Input: part model. Units: mm. Frame: model coordinates. Face numbers are marked on the shaded views. A direction names the side the tool comes from. Round coordinates to 2 decimals unless told otherwise and drop trailing zeros. Loops run counter-clockwise (first coordinate to the right, second up) from the corner with the lowest first, then second, coordinate; pieces in that order, holes last. Notation, with made-up numbers: (10.5, 80.25) -> (42.5, 80.25) arc R16 ccw to (42.5, 110.25) -> close; hole circle Ø1 at (16, 30.5). An arc over 180 degrees is marked (long way). Answer in a Markdown table with one row per item. Add a question column.
Q1. Ray query, L1, parallel to X at y = -20.25, z = 0.25; L2, parallel to X at y = -4, z = -2.25; L3, parallel to Z at x = 2.25, y = -18.5. Return the intervals inside material, ascending. Write a range as from..to.
Q2. Section B-B, the plane x = 4. Output: boundary loops of the cut face in (y, z), and give its area (3 significant figures).
Q3. Mould query, pull axis Z, two halves, no side actions, for the marked faces 3, 4 and 5. Classes: pulls with the +Z half, pulls with the -Z half, needs draft (parallel to the pull), parting line crosses it, or undercut.
Q4. Section A-A, the plane z = 2.75. Output: boundary loops of the cut face in (x, y).
Q5. Section D-D, the plane z = -8. Output: boundary loops of the cut face in (x, y).
Q6. Reachability of the marked faces 1 and 2 from +Z, -Z, +X, -X, +Y, -Y: full face, straight path, thin tool, end or side. Return the list, or none.
Q7. Pin query (flat end, axial travel): pin 1 (2 mm diameter, centred on y = -16.5, z = -3, fed in from +X); pin 2 (5 mm diameter, centred on x = -3, y = -12.5, fed in from -Z); pin 3 (1.7 mm diameter, centred on y = -2, z = 1, fed in from -X); pin 4 (4 mm diameter, centred on x = -1, z = -2.5, fed in from +Y). Return the tip coordinate at first contact, or that it passes through.
```python
from build123d import *

# Parameters (mm, degrees)
F0_R     = 9.525
F1_DEPTH = 25.4
F3_DEPTH = 25.401
F4_DEPTH = 5.5499


with BuildPart() as f1:
    # F0 (on Front) → F1 (new body)
    with BuildSketch(Plane.XZ):
        Circle(F0_R)
    extrude(amount=F1_DEPTH)

    # F2 (on Front) → F3 (cut, through all)
    with BuildSketch(Plane.XZ):
        with BuildLine():
            ThreePointArc((4.7625, 0), (3.367596, 3.367596), (0, 4.7625))
            ThreePointArc((0, 4.7625), (-3.367596, 3.367596), (-4.7625, 0))
            ThreePointArc((-4.7625, 0), (-3.367596, -3.367596), (0, -4.7625))
            ThreePointArc((0, -4.7625), (3.367596, -3.367596), (4.7625, 0))
        make_face()
    extrude(amount=F3_DEPTH, mode=Mode.SUBTRACT)

    # F2 (on Front) → F4 (cut, symmetric)
    with BuildSketch(Plane.XZ):
        with BuildLine():
            Line((0, 4.7625), (-4.7625, 4.7625))
            Line((-4.7625, 4.7625), (-4.7625, 0))
            ThreePointArc((-4.7625, 0), (-3.367596, 3.367596), (0, 4.7625))
        make_face()
        with BuildLine():
            Line((4.7625, 4.7625), (0, 4.7625))
            ThreePointArc((0, 4.7625), (3.367596, 3.367596), (4.7625, 0))
            Line((4.7625, 0), (4.7625, 4.7625))
        make_face()
        with BuildLine():
            ThreePointArc((0, -4.7625), (-3.367596, -3.367596), (-4.7625, 0))
            Line((-4.7625, 0), (-4.7625, -4.7625))
            Line((-4.7625, -4.7625), (0, -4.7625))
        make_face()
        with BuildLine():
            Line((4.7625, -4.7625), (4.7625, 0))
            ThreePointArc((4.7625, 0), (3.367596, -3.367596), (0, -4.7625))
            Line((0, -4.7625), (4.7625, -4.7625))
        make_face()
    extrude(amount=F4_DEPTH, both=True, mode=Mode.SUBTRACT)


solid = f1.part
```
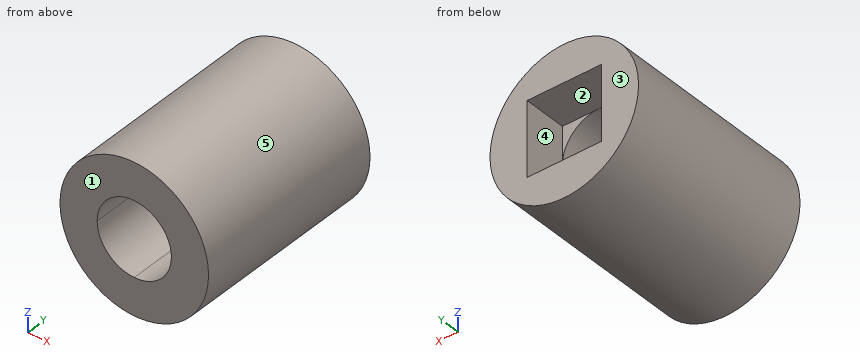
Answer block:
| question | item | result |
|---|---|---|
| 1 | L1 | -9.52..-4.76, 4.76..9.52 |
| 1 | L2 | -9.26..-4.76, 4.76..9.26 |
| 1 | L3 | -9.26..-4.2, 4.2..9.26 |
| 2 | outline | (-25.4, -8.64) -> (0, -8.64) -> (0, -4.76) -> (-5.55, -4.76) -> (-5.55, -2.58) -> (-25.4, -2.58) -> close; (-25.4, 2.58) -> (-5.55, 2.58) -> (-5.55, 4.76) -> (0, 4.76) -> (0, 8.64) -> (-25.4, 8.64) -> close |
| 2 | area | 284 mm^2 |
| 3 | face 3 | needs draft |
| 3 | face 4 | undercut |
| 3 | face 5 | parting line crosses it |
| 4 | outline | (-9.12, -25.4) -> (-3.89, -25.4) -> (-3.89, -5.55) -> (-4.76, -5.55) -> (-4.76, 0) -> (-9.12, 0) -> close; (3.89, -25.4) -> (9.12, -25.4) -> (9.12, 0) -> (4.76, 0) -> (4.76, -5.55) -> (3.89, -5.55) -> close |
| 5 | outline | (-5.17, -25.4) -> (5.17, -25.4) -> (5.17, 0) -> (-5.17, 0) -> close |
| 6 | face 1 | +Z, -Z, +X, -X, -Y |
| 6 | face 2 | +Y |
| 7 | pin 1 | x = 9.31 |
| 7 | pin 2 | z = -9.51 |
| 7 | pin 3 | x = -9.52 |
| 7 | pin 4 | through |
